Geometry check sheet. Reference: the model listing, model coordinates, mm. A direction names the side the tool comes from. Coordinates: 2 decimals unless noted, no trailing zeros. Order: outer loops, then holes, each group sorted by start corner. A loop starts at its lowest first (then second) coordinate and runs counter-clockwise, first axis right, second up. Notation, with made-up numbers: (12, -28.5) -> (58, -28.5) arc R26 cw to (58, -7.5) -> close; hole circle Ø8 at (46.25, 26.25). An arc over 180 degrees is marked (long way). Answer in a Markdown table with one row per item. Add a question column.
Autodesk Inventor part; units mm, degrees
ref_plane "作業平面1" through (0, 48.5, 0) normal (0, 1, 0) x (1, 0, 0)
ref_plane "YZ Plane" through (0, 0, 0) normal (1, 0, 0) x (0, 1, 0)
ref_plane "XZ Plane" through (0, 0, 0) normal (0, 1, 0) x (-1, 0, 0)
sketch "スケッチ1" plane through (0, 0, 0) normal (0, 1, 0) x (-1, 0, 0)
  line L0 (8.2272, -4.75) -> (0, 0)
  line L1 (0, 0) -> (-10.8031, -18.7115)
  line L2 (-10.8031, -18.7115) -> (-5.3183, -28.2115)
  line L3 (-5.3183, -28.2115) -> (8.2272, -4.75)
  line L4 (31.5369, 0) -> (-17.8598, 0)
  line L5 (0, 0) -> (19.1969, 33.25)
  line L6 (19.1969, 33.25) -> (24.4803, 30.1996) construction
  line L7 (5.1962, -3) -> (1.9462, -8.6292)
  line L8 (1.9462, -8.6292) -> (4.9772, -10.3792)
  dimension "d0" = 9.5
  dimension "d2" = 60
  dimension "d3" = 60
  dimension "d4" = 60
  dimension "d8" = 38
  dimension "d9" = 3.5
  dimension "d10" = 6.5
extrude "押し出し1" add sketch "スケッチ1" along normal blind 97 contours L7 L8 L3 L2 L1 L0
sketch "スケッチ2" plane through (-5.1962, 0, -3) normal (-0.866, 0, -0.5) x (-0.5, 0, 0.866)
  circle A0 centre (-3, 3.5) radius 3
  line L0 (-6.5, 0) -> (0, 0)
  line L1 (0, 0) -> (0, 97)
  circle A1 centre (-3, 3.5) radius 1.35
  dimension "d12" = 6
  dimension "d13" = 3.5
  dimension "d14" = 2.7
extrude "押し出し2" cut sketch "スケッチ2" against normal through all contours A1
sketch "スケッチ3" plane through (-5.1962, 0, -3) normal (-0.866, 0, -0.5) x (-0.5, 0, 0.866)
  circle A0 centre (-3, 3.5) radius 1.35
  circle A1 centre (-3, 3.5) radius 2.25
  point P0 (0, 0)
  dimension "d17" = 4.5
extrude "押し出し3" add sketch "スケッチ3" along normal blind 0.5
sketch "スケッチ4" plane through (0, 0, 0) normal (-0.5, 0, 0.866) x (0.866, 0, 0.5)
  circle A0 centre (-3.5, 10.5) radius 3
  line L0 (-6, 0) -> (-6, 97)
  line L1 (-6, 7) -> (0, 7)
  line L2 (-6, 0) -> (0, 0)
  line L3 (-9.5, 0) -> (-6, 0)
  line L4 (-6.5, 0) -> (-6.5, 11.2829)
  circle A1 centre (-3.5, 10.5) radius 1.35
  dimension "d20" = 6
  dimension "d21" = 7
  dimension "d22" = 3.5
  dimension "d23" = 0.5
  dimension "d24" = 2.7
extrude "押し出し4" cut sketch "スケッチ4" against normal blind 5 contours A1
sketch "スケッチ5" plane through (0, 0, 0) normal (-0.5, 0, 0.866) x (0.866, 0, 0.5)
  circle A0 centre (-3.5, 10.5) radius 1.35
  circle A1 centre (-3.5, 10.5) radius 2.25
  point P0 (0, 0)
  dimension "d27" = 4.5
extrude "押し出し5" add sketch "スケッチ5" along normal blind 0.2
pattern_linear "矩形状パターン1" count 4 spacing 27.6667 along (0, 1, 0) of "押し出し2", "押し出し3", "押し出し4", "押し出し5"
sketch "スケッチ6" plane through (-4.9772, 0, -10.3792) normal (-0.866, 0, -0.5) x (-0.5, 0, 0.866)
  line L0 (-20.591, 0) -> (-20.591, 97)
  line L1 (-20.591, 96) -> (-1.091, 96)
  line L2 (-1.091, 96) -> (-1.091, 81.4)
  line L3 (-1.091, 81.4) -> (-20.591, 81.4)
  line L4 (-20.591, 81.4) -> (-20.591, 96)
  line L5 (-20.591, 97) -> (0, 97)
  line L6 (-20.591, 96) -> (-1.091, 96)
  line L7 (-1.091, 96) -> (-1.091, 97)
  line L8 (-1.091, 97) -> (-20.591, 97)
  line L9 (-20.591, 97) -> (-20.591, 96)
  circle A0 centre (-15.591, 89.1) radius 0.85
  circle A1 centre (-6.091, 89.1) radius 0.85
  line L10 (-10.841, 81.4) -> (-10.841, 96)
  point P0 (6.5, 0)
  point P1 (-1.091, 96)
  dimension "d33" = 19.5
  dimension "d34" = 14.6
  dimension "d35" = 1
  dimension "d36" = 1.7
  dimension "d37" = 6.9
  dimension "d38" = 9.5
extrude "押し出し6" cut sketch "スケッチ6" against normal through all contours A0 | A1
sketch "スケッチ8" plane through (0, 97, 0) normal (0, 1, 0) x (1, 0, 0)
  line L0 (4.5139, 11.4183) -> (2.8684, 8.5683)
  line L1 (2.8684, 8.5683) -> (-0.4225, 8.5683)
  line L2 (-0.4225, 8.5683) -> (-2.0679, 11.4183)
  line L3 (-2.0679, 11.4183) -> (-0.4225, 14.2683)
  line L4 (-0.4225, 14.2683) -> (2.8684, 14.2683)
  line L5 (2.8684, 14.2683) -> (4.5139, 11.4183)
  line L6 (6.9637, 15.6615) -> (3.6728, 15.6615)
  line L7 (3.6728, 15.6615) -> (2.0274, 18.5115)
  line L8 (2.0274, 18.5115) -> (3.6728, 21.3615)
  line L9 (3.6728, 21.3615) -> (6.9637, 21.3615)
  line L10 (6.9637, 21.3615) -> (8.6092, 18.5115)
  line L11 (8.6092, 18.5115) -> (6.9637, 15.6615)
  line L12 (5.3183, 28.2115) -> (-4.9772, 10.3792)
  line L13 (10.8031, 18.7115) -> (5.3183, 28.2115)
  line L14 (-4.9772, 10.3792) -> (-1.9462, 8.6292)
  line L15 (-0.4225, 8.5683) -> (3.6046, 6.2433)
  line L16 (0, 0) -> (10.8031, 18.7115)
  line L17 (2.8684, 14.2683) -> (6.8954, 11.9433)
  line L18 (3.6728, 15.6615) -> (7.6998, 13.3365)
  line L19 (6.9637, 21.3615) -> (11.0441, 19.0057)
  circle A0 centre (1.223, 11.4183) radius 1.6
  circle A1 centre (5.3183, 18.5115) radius 1.6
  point P0 (10.4278, 19.3615)
  dimension "d47" = 5.7
  dimension "d48" = 2
  dimension "d49" = 2
  dimension "d50" = 4
  dimension "d51" = 3.2
  dimension "d52" = 3.2
extrude "押し出し8" cut sketch "スケッチ8" against normal blind 15 contours A0 | A1
extrude "押し出し9" cut sketch "スケッチ8" against normal blind 6
extrude "押し出し10" add sketch "スケッチ8" against normal blind 3
ref_plane "作業平面1" through (0, 48.5, 0) normal (0, 1, 0) x (1, 0, 0)
mirror "ミラー1" about plane through (0, 48.5, 0) normal (0, 1, 0) of "押し出し8", "押し出し9", "押し出し10"
properties part number "base_bearingpole_side"
(1) Scan lines: line 1 along Y through (x, z) = (-0.75, -12.5); line 2 along Y through (x, z) = (-2.25, -2); line 3 along Y through (x, z) = (5.5, -10.5). Record each from-to range of solid material in increasing order.
(2) Cross-section at B-B (z = -26). Enter the section's corners in (x, y), plus the area to 3 significant figures.
(3) Cross-section at A-A (y = 42.5). Enter the section's corners in (x, z), plus the area to 3 significant figures.
(4) Access from +Z, -Z, +X, -X, +Y, -Y to the whole of each face (thin tool, end or side, straight path). Record for faces 1 (the face through (5.11, 95.521, -20.098)), 2 (the face through (1.6, 4.5, -7.4)), 3 (the face through (7, 6, -17)).
(5) Go/stop test with flat-tipped pins: P1, Ø1, axis at x = 5, z = -19, coming from the +Y side; P2, Ø1.5, axis at x = 5, y = 4.5, coming from the +Z side; P3, Ø1.9, axis at x = 1.22, z = -11.42, coming from the -Y side. Record where each tip stops, or that it passes through.
Checks:
| question | item | result |
|---|---|---|
| 1 | line 1 | 0 to 3, 6 to 91, 94 to 97 |
| 1 | line 2 | 0 to 9.27, 11.73 to 36.93, 39.4 to 64.6, 67.07 to 92.27, 94.73 to 97 |
| 1 | line 3 | 0 to 3, 6 to 88.7, 89.5 to 91, 94 to 97 |
| 2 | outline | (4.04, 0) -> (6.6, 0) -> (6.6, 97) -> (4.04, 97) -> close |
| 2 | area | 248 mm² |
| 3 | outline | (-5.2, -3) -> (-1.95, -8.63) -> (-4.98, -10.38) -> (5.32, -28.21) -> (10.8, -18.71) -> (0, 0) -> close |
| 3 | area | 209 mm² |
| 4 | face 1 | +Y |
| 4 | face 2 | +X |
| 4 | face 3 | none |
| 5 | P1 | y = 82 |
| 5 | P2 | z = -12.6 |
| 5 | P3 | y = 15 |
